from build123d import *

# Parameters (mm, degrees)
F1_DEPTH = 38.1
F2_DEPTH = 19.05


# Not quite as in the source:
# - a length typed as a fraction of an inch, garbled in the dataset ("3 / 203.2 mm" for 3/8 in), is restored


with BuildPart() as f1:
    # F0 (on Front) → F1 (new body)
    with BuildSketch(Plane.XZ):
        Polygon((-63.5, 9.3406075202), (-63.5, -22.4093924798), (63.5, -22.4093924798), (63.5, 9.3406075202), (0, 9.3406075202), align=None)
    extrude(amount=F1_DEPTH)

    # F0 (on Front) → F2 (join)
    with BuildSketch(Plane.XZ):
        Polygon((-63.5, 41.0906075202), (-63.5, 9.3406075202), (0, 9.3406075202), align=None)
        Polygon((0, 9.3406075202), (63.5, 9.3406075202), (0, 41.0906075202), align=None)
    extrude(amount=F2_DEPTH)


solid = f1.part
The listing builds one solid part. Answer for the finished solid, in the listing's coordinates (mm). A direction names the side the tool comes from. Round coordinates to 2 decimals unless told otherwise and drop trailing zeros. Write each loop counter-clockwise with the first axis right and the second up, starting at its lowest first coordinate (ties: lowest second). Pieces come first, ordered by that corner, then holes. Notation, with made-up numbers: M 49,-24 L 103,-24 A25 cw 103,5 Z; hole C 32,75.25 d4. An arc over 180 degrees is marked long. Write each question's results on one line, items separated by ' | '. Start each with the question number.
(1) The part is cut by section C-C, the plane x = -24.5. Write down the section's boundary in (y, z).
(2) The part is cut by section B-B, the plane y = -4. Write down the section's boundary in (x, z), and give its area (3 significant figures).
(3) The part is cut by section A-A, the plane z = 15.5. Write down the section's boundary in (x, y), and give its area (3 significant figures).
(4) For faces 4 (the flat face through (-1, -38.1, -6)), 5 (the flat face through (0, -9, 25)), 6 (the flat face through (17, -19.05, 18)), determine the directions among +Z, -Z, +X, -X, +Y, -Y from which every point of the face is accessible in a straight line to the end or side of a thin tool.
(5) Each of these flat-tipped pins is pushed along its axis until it touches: P1, Ø10, axis at x = 43.5, y = -7.5, coming from the +Z side; P2, Ø10, axis at x = 31, y = -15.5, coming from the +Z side; P3, Ø1.5, axis at x = 29, y = -20.5, coming from the +Z side; P4, Ø1.5, axis at x = 9, z = 34, coming from the +Y side. Where does it stop, or does it pass through?
(6) Determine the mould class of faces 1 (the flat face through (32.194, -9.392, 24.993)), 2 (the flat face through (-1, -19, -22.409)), 3 (the flat face through (-31.306, -9.392, 24.993)) for opening direction X: +X half, -X half, draft (parallel to the pull), parting line (faces both ways), or undercut.
(7) Find the intervals of material crossed by line 1 (X direction, y = -11.5, z = 37.5); line 2 (Z direction, x = -31, y = -34.5); line 3 (Y direction, x = -57, z = 17.5), in increasing order.
(8) The part is cut by section D-D, the plane z = 36. Write down the section's boundary in (x, y).
Worked answers:
1) outline: M -38.1,-22.41 L 0,-22.41 L 0,21.59 L -19.05,21.59 L -19.05,9.34 L -38.1,9.34 Z
2) outline: M -63.5,-22.41 L 63.5,-22.41 L 63.5,9.34 L 0,41.09 L 0,9.34 L -63.5,41.09 Z | area: 6,050 mm²
3) outline: M -63.5,-19.05 L -12.32,-19.05 L -12.32,0 L -63.5,0 Z; M 0,-19.05 L 51.18,-19.05 L 51.18,0 L 0,0 Z | area: 1,950 mm²
4) face 4: +Z, -Z, +X, -X, -Y | face 5: +Z, +Y, -Y | face 6: +Z, +X, -X, -Y
5) P1: stops at z = 21.84 | P2: stops at z = 28.09 | P3: stops at z = 9.34 | P4: stops at y = 0
6) face 1: +X half | face 2: draft | face 3: undercut
7) line 1: x = -63.5 to -56.32, 0 to 7.18 | line 2: z = -22.41 to 9.34 | line 3: y = -19.05 to 0
8) outline: M -63.5,-19.05 L -53.32,-19.05 L -53.32,0 L -63.5,0 Z; M 0,-19.05 L 10.18,-19.05 L 10.18,0 L 0,0 Z
